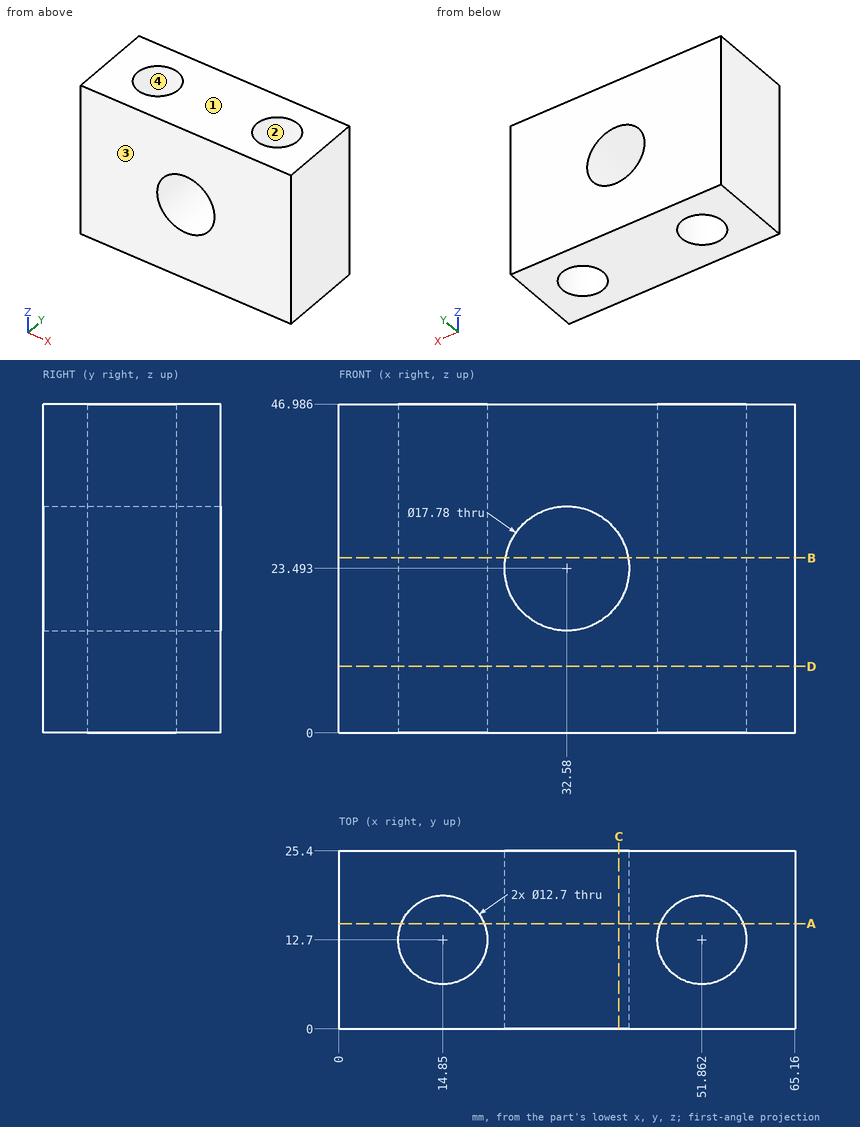
Geometry check sheet. Reference: drawing and pictorial views, mm from the part's lowest x, y, z. Coordinates: 2 decimals unless noted, no trailing zeros. Loops run counter-clockwise (first coordinate to the right, second up) from the corner with the lowest first, then second, coordinate; pieces in that order, holes last. Notation, with made-up numbers: (46.5, 31) - (88.5, 31) arc R26 ccw to (88.5, 69) - close; hole circle Ø3 at (39.5, 60.25). An arc over 180 degrees is marked (long way). Return JSON: item names as keys, results as strings.
1. Section check D-D, the plane z = 9.5. Record the boundary of the cut face in (x, y).
Established:
{"outline": "(0, 0) - (65.16, 0) - (65.16, 25.4) - (0, 25.4) - close; hole circle Ø12.7 at (14.85, 12.7); hole circle Ø12.7 at (51.86, 12.7)"}
2. Section check A-A, the plane y = 15. Record the boundary of the cut face in (x, z), then the cut area to 3 significant figures.
Established:
{"outline": "(0, 0) - (8.93, 0) - (8.93, 46.99) - (0, 46.99) - close; (20.77, 0) - (45.94, 0) - (45.94, 46.99) - (20.77, 46.99) - close; (57.78, 0) - (65.16, 0) - (65.16, 46.99) - (57.78, 46.99) - close; hole circle Ø17.78 at (32.58, 23.49)", "area": "1,700 mm2"}
3. Thickness scan on L1, parallel to X at y = 9, z = 9.5 (1 decimal); L2, parallel to X at y = 14.5, z = 39; L3, parallel to Y at x = 13.5, z = 15.5 (1 decimal). Record the ranges inside material, lowest first.
Established:
{"L1": "x = 0 to 9.7, 20 to 46.7, 57 to 65.2", "L2": "x = 0 to 8.76, 20.94 to 45.77, 57.95 to 65.16", "L3": "y = 0 to 6.5, 18.9 to 25.4"}
4. Section check C-C, the plane x = 40. Record the boundary of the cut face in (y, z).
Established:
{"outline": "(0, 0) - (25.4, 0) - (25.4, 18.6) - (0, 18.6) - close; (0, 28.39) - (25.4, 28.39) - (25.4, 46.99) - (0, 46.99) - close"}
5. Section check B-B, the plane z = 25. Record the boundary of the cut face in (x, y).
Established:
{"outline": "(0, 0) - (23.82, 0) - (23.82, 25.4) - (0, 25.4) - close; (41.34, 0) - (65.16, 0) - (65.16, 25.4) - (41.34, 25.4) - close; hole circle Ø12.7 at (14.85, 12.7); hole circle Ø12.7 at (51.86, 12.7)"}
6. Mould release check, pull along Y, two halves, no side actions. Record for the marked faces 1, 2, 3 and 4: +Y half, -Y half, draft (parallel to the pull), parting line (faces both ways), or undercut.
Established:
{"face 1": "draft", "face 2": "undercut", "face 3": "-Y half", "face 4": "undercut"}
